The listing builds one solid part. Answer for the finished solid, in the listing's coordinates (mm). Face numbers are marked on the shaded views. A direction names the side the tool comes from. Give positions to 0.01 mm unless a question says otherwise; leave off trailing zeros. Order: outer loops, then holes, each group sorted by start corner. A loop starts at its lowest first (then second) coordinate and runs counter-clockwise, first axis right, second up. Notation, with made-up numbers: (41.25, -9) - (56.25, -9) arc R8 cw to (56.25, 4) - close; hole circle Ø7 at (3.5, 13). An arc over 180 degrees is marked (long way). Answer as a JSON object with one key per item and string values. Group by question number.
Q1. For the marked faces 1 and 2, determine the directions among +Z, -Z, +X, -X, +Y, -Y from which every point of the face is accessible in a straight line to the end or side of a thin tool.
Q2. Given pin 1 (3 mm diameter, centred on x = -10.5, y = 19.5, fed in from +Z); pin 2 (11.5 mm diameter, centred on x = -6, z = 39, fed in from -Y), each flat-ended and moving along its own axis, determine where each tip first touches the part or whether it passes through.
Q3. A cutting plane is placed at C-C, the plane y = 17.25. Give the vertices of the cut face in (x, z), and give its area (3 significant figures).
Q4. A cutting plane is placed at B-B, the plane x = -13.5. Give the vertices of the cut face in (y, z).
Q5. A cutting plane is placed at D-D, the plane z = 42.5. Give the vertices of the cut face in (x, y), and give its area (3 significant figures).
Q6. Consider line 1 (Y direction, x = 6.5, z = 53); line 2 (Z direction, x = -16.5, y = 24); line 3 (Z direction, x = 12.5, y = 30). Determine where each line is inside the solid, lowest interval first.
Q7. A cutting plane is placed at A-A, the plane z = 53. Give the vertices of the cut face in (x, y), and give its area (3 significant figures).
from build123d import *

# Parameters (mm, degrees)
SKETCH_1_W          = 38
SKETCH_1_H          = 38
EXTRUDE_1_DEPTH     = 8
SKETCH_2_W          = 38
SKETCH_2_H          = 6
EXTRUDE_2_DEPTH     = 50
SKETCH_3_W          = 38
SKETCH_3_H          = 16
CUT_EXTRUDE_1_DEPTH = 10
SKETCH_4_R          = 3.2
CUT_EXTRUDE_2_DEPTH = 10
SKETCH_5_R          = 1.6
CUT_EXTRUDE_3_DEPTH = 10


with BuildPart() as part:
    # 草图1 → 拉伸1 (new body)
    with BuildSketch(Plane.XY):
        with Locations((-0.319940249, 13.481833206)):
            Rectangle(SKETCH_1_W, SKETCH_1_H)
    extrude(amount=EXTRUDE_1_DEPTH)

    # 草图2 → 拉伸2 (add)
    with BuildSketch(Plane.XY.offset(8)):
        with Locations((-0.319940249, 29.481833206)):
            Rectangle(SKETCH_2_W, SKETCH_2_H)
    extrude(amount=EXTRUDE_2_DEPTH)

    # 草图3 → 切除-拉伸1 (cut)
    with BuildSketch(Plane.XY.offset(8)):
        with Locations((-0.319940249, 2.481833206)):
            Rectangle(SKETCH_3_W, SKETCH_3_H)
    extrude(amount=-CUT_EXTRUDE_1_DEPTH, mode=Mode.SUBTRACT)

    # 草图4 → 切除-拉伸2 (cut)
    with BuildSketch(Plane.XY.offset(8)):
        with Locations((-12.819940249, 18.481833206)):
            Circle(SKETCH_4_R)
        with Locations((12.180059751, 18.481833206)):
            Circle(SKETCH_4_R)
    extrude(amount=-CUT_EXTRUDE_2_DEPTH, mode=Mode.SUBTRACT)

    # 草图5 → 切除-拉伸3 (cut)
    with BuildSketch(Plane.XZ.offset(-26.481833206)):
        with Locations(Location((12.180059751, 53, 0), (0, 0, 270))):
            Circle(SKETCH_5_R)
        with Locations(Location((-12.819940249, 53, 0), (0, 0, 270))):
            Circle(SKETCH_5_R)
    extrude(amount=-CUT_EXTRUDE_3_DEPTH, mode=Mode.SUBTRACT)


solid = part.part
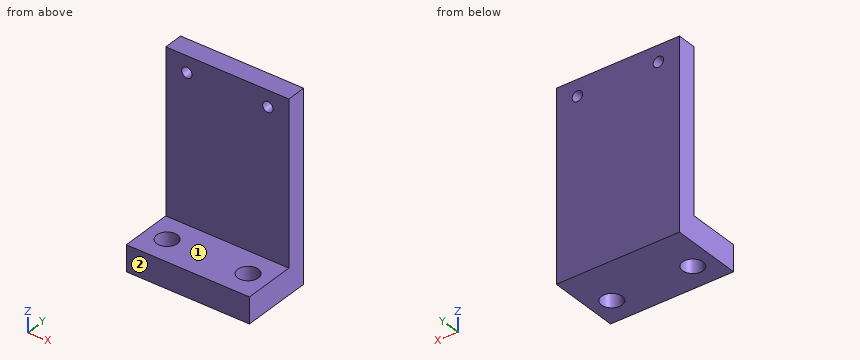
Reply:
{
 "1": {"face 1": "+Z, +X, -X, -Y", "face 2": "+Z, -Z, +X, -X, -Y"},
 "2": {"pin 1": "stops at z = 8", "pin 2": "stops at y = 26.48"},
 "3": {"outline": "(-19.32, 0) - (-15.77, 0) - (-15.77, 8) - (-19.32, 8) - close; (-9.87, 0) - (9.23, 0) - (9.23, 8) - (-9.87, 8) - close; (15.13, 0) - (18.68, 0) - (18.68, 8) - (15.13, 8) - close", "area": "209 mm^2"},
 "4": {"outline": "(10.48, 0) - (15.35, 0) - (15.35, 8) - (10.48, 8) - close; (21.61, 0) - (32.48, 0) - (32.48, 51.55) - (26.48, 51.55) - (26.48, 8) - (21.61, 8) - close; (26.48, 54.45) - (32.48, 54.45) - (32.48, 58) - (26.48, 58) - close"},
 "5": {"outline": "(-19.32, 26.48) - (18.68, 26.48) - (18.68, 32.48) - (-19.32, 32.48) - close", "area": "228 mm^2"},
 "6": {"line 1": "y = 26.48 to 32.48", "line 2": "z = 0 to 8", "line 3": "z = 0 to 51.43, 54.57 to 58"},
 "7": {"outline": "(-19.32, 26.48) - (-14.42, 26.48) - (-14.42, 32.48) - (-19.32, 32.48) - close; (-11.22, 26.48) - (10.58, 26.48) - (10.58, 32.48) - (-11.22, 32.48) - close; (13.78, 26.48) - (18.68, 26.48) - (18.68, 32.48) - (13.78, 32.48) - close", "area": "190 mm^2"}
}
